```python
from build123d import *
from build123d.topology import SkipClean

# Parameters (mm, degrees)
SKETCH1_R           = 4
SKETCH1_R_2         = 12.5
SKETCH1_R_3         = 1.55
SKETCH1_W           = 10
SKETCH1_H           = 3
BOSS_EXTRUDE1_DEPTH = 5
BOSS_EXTRUDE2_START = 3
SKETCH2_R           = 17
BOSS_EXTRUDE2_DEPTH = 3
SKETCH3_R           = 1.55
SKETCH3_R_2         = 1
CUT_EXTRUDE1_DEPTH  = 8
SKETCH4_R           = 3
SKETCH4_R_2         = 2.2
CUT_EXTRUDE2_DEPTH  = 4.5
SKETCH5_R           = 8
CUT_EXTRUDE3_DEPTH  = 5


with BuildPart() as part:
    # Sketch1 → Boss-Extrude1 (new body)
    with BuildSketch(Plane.XY):
        with BuildLine():
            Line((-25, 0), (25, 0))
            Line((25, 0), (25, 10))
            Line((25, 10), (17, 150))
            ThreePointArc((17, 150), (0, 167), (-17, 150))
            Line((-17, 150), (-25, 10))
            Line((-25, 10), (-25, 0))
        make_face()
        with Locations((0, 150)):
            Circle(SKETCH1_R, mode=Mode.SUBTRACT)
        with Locations((0, 90)):
            Circle(SKETCH1_R_2, mode=Mode.SUBTRACT)
        with Locations((-8, 6.5)):
            Circle(SKETCH1_R_3, mode=Mode.SUBTRACT)
        with Locations((-16, 3.5)):
            Circle(SKETCH1_R_3, mode=Mode.SUBTRACT)
        with Locations((8, 6.5)):
            Circle(SKETCH1_R_3, mode=Mode.SUBTRACT)
        with Locations((16, 3.5)):
            Circle(SKETCH1_R_3, mode=Mode.SUBTRACT)
        with Locations((-15.5, 71.5)):
            Circle(SKETCH1_R_3, mode=Mode.SUBTRACT)
        with Locations((15.5, 71.5)):
            Circle(SKETCH1_R_3, mode=Mode.SUBTRACT)
        with Locations((0, 70)):
            Rectangle(SKETCH1_W, SKETCH1_H, mode=Mode.SUBTRACT)
    extrude(amount=BOSS_EXTRUDE1_DEPTH)

    # Sketch2 → Boss-Extrude2 (add)
    with SkipClean():  # the faces are left unmerged after this step: merging them gives an invalid solid
        with BuildSketch(Plane(origin=(0, 0, 0), x_dir=(-1, 0, 0), z_dir=(0, 0, -1)).offset(BOSS_EXTRUDE2_START)):
            with Locations((0, 150)):
                Circle(SKETCH2_R)
        extrude(amount=-BOSS_EXTRUDE2_DEPTH)

    # Sketch3 → Cut-Extrude1 (cut)
    with SkipClean():  # the faces are left unmerged after this step: merging them gives an invalid solid
        with BuildSketch(Plane.XY.offset(5)):
            with Locations((-12.5, 150)):
                Circle(SKETCH3_R)
            with Locations((0, 162.5)):
                Circle(SKETCH3_R)
            with Locations((12.5, 150)):
                Circle(SKETCH3_R)
            with Locations((0, 137.5)):
                Circle(SKETCH3_R)
            with Locations((8.980256121, 158.980256121)):
                Circle(SKETCH3_R_2)
            with Locations((8.980256121, 141.019743879)):
                Circle(SKETCH3_R_2)
            with Locations((-8.980256121, 141.019743879)):
                Circle(SKETCH3_R_2)
            with Locations((-8.980256121, 158.980256121)):
                Circle(SKETCH3_R_2)
        extrude(amount=-CUT_EXTRUDE1_DEPTH, mode=Mode.SUBTRACT)

    # Sketch4 → Cut-Extrude2 (cut)
    with SkipClean():  # the faces are left unmerged after this step: merging them gives an invalid solid
        with BuildSketch(Plane.XY.offset(5)):
            with Locations((-12.5, 150)):
                Circle(SKETCH4_R)
            with Locations((0, 162.5)):
                Circle(SKETCH4_R)
            with Locations((12.5, 150)):
                Circle(SKETCH4_R)
            with Locations((0, 137.5)):
                Circle(SKETCH4_R)
            with Locations((-8.980256121, 158.980256121)):
                Circle(SKETCH4_R_2)
            with Locations((8.980256121, 158.980256121)):
                Circle(SKETCH4_R_2)
            with Locations((8.980256121, 141.019743879)):
                Circle(SKETCH4_R_2)
            with Locations((-8.980256121, 141.019743879)):
                Circle(SKETCH4_R_2)
        extrude(amount=-CUT_EXTRUDE2_DEPTH, mode=Mode.SUBTRACT)

    # Sketch5 → Cut-Extrude3 (cut)
    with SkipClean():  # the faces are left unmerged after this step: merging them gives an invalid solid
        with BuildSketch(Plane(origin=(0, 0, -3), x_dir=(-1, 0, 0), z_dir=(0, 0, -1))):
            with Locations((0, 150)):
                Circle(SKETCH5_R)
        extrude(amount=-CUT_EXTRUDE3_DEPTH, mode=Mode.SUBTRACT)


solid = part.part
```
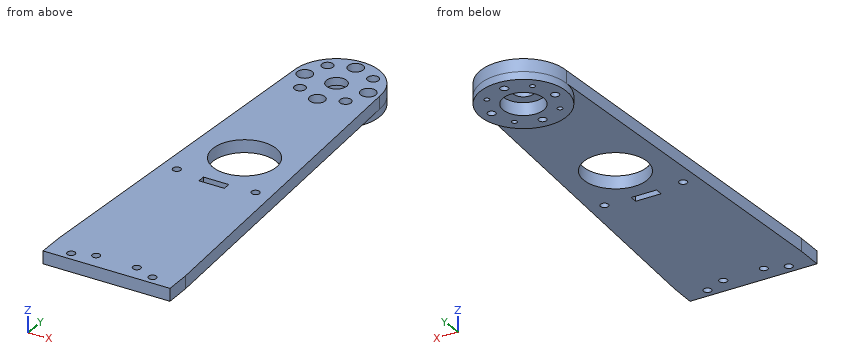
Model file for the job. Use its own axes, mm. Coordinates: 2 decimals unless noted, no trailing zeros. Order: outer loops, then holes, each group sorted by start corner. A loop starts at its lowest first (then second) coordinate and runs counter-clockwise, first axis right, second up. Notation, with made-up numbers: (5, -1) - (54, -1) arc R23 cw to (54, 18) - close; hole circle Ø11 at (50, -14). An arc over 180 degrees is marked (long way). Return JSON: item names as keys, results as strings. Group by question number.
1) Saw through at B-B, the plane x = 0. Count the separate pieces of the cut face and the enclosed holes in it, plus the area to 3 significant figures.
2) Saw through at D-D, the plane x = 20. Write the cut outline in (y, z).
3) Saw through at A-A, the plane y = 3.5. Write the cut outline in (x, z).
4) Probe line 1 (Y direction, x = 0, z = 3.2); line 2 (Y direction, x = 0.5, z = 1.75); line 3 (X direction, y = 151.5, z = 1.5). List the from-to ranges inside material, lowest first. Write a range as from..to.
5) Flat gauge pins, fed straight in: P1, Ø3.5, axis at x = 15.5, y = 71.5, coming from the -Z side; P2, Ø2, axis at y = 107.5, z = 3.5, coming from the -X side; P3, Ø1.3, axis at x = 10, y = 140, coming from the +Z side; P4, Ø1.8, axis at x = 8.98, y = 158.98, coming from the +Z side. Where does each tip first touch, or does it go through?
Values found:
{
 "1": {"separate pieces": "6", "enclosed holes": "0", "area": "617 mm²"},
 "2": {"outline": "(0, 0) - (97.5, 0) - (97.5, 5) - (0, 5) - close"},
 "3": {"outline": "(-25, 0) - (-17.55, 0) - (-17.55, 5) - (-25, 5) - close; (-14.45, 0) - (14.45, 0) - (14.45, 5) - (-14.45, 5) - close; (17.55, 0) - (25, 0) - (25, 5) - (17.55, 5) - close"},
 "4": {"line 1": "y = 0..68.5, 71.5..77.5, 102.5..134.5, 140.5..146, 154..159.5, 165.5..167", "line 2": "y = 0..68.5, 71.5..77.51, 102.49..134.54, 140.46..142.02, 157.98..159.54, 165.46..166.99", "line 3": "x = -16.93..-15.1, -9.9..-7.86, 7.86..9.9, 15.1..16.93"},
 "5": {"P1": "stops at z = 0", "P2": "stops at x = -19.49", "P3": "stops at z = 0.5", "P4": "passes through"}
}
